Verification items for this drawing (mm, ordinates from the low corner). A direction names the side the tool comes from. Coordinates: 2 decimals unless noted, no trailing zeros. Loops run counter-clockwise (first coordinate to the right, second up) from the corner with the lowest first, then second, coordinate; pieces in that order, holes last.
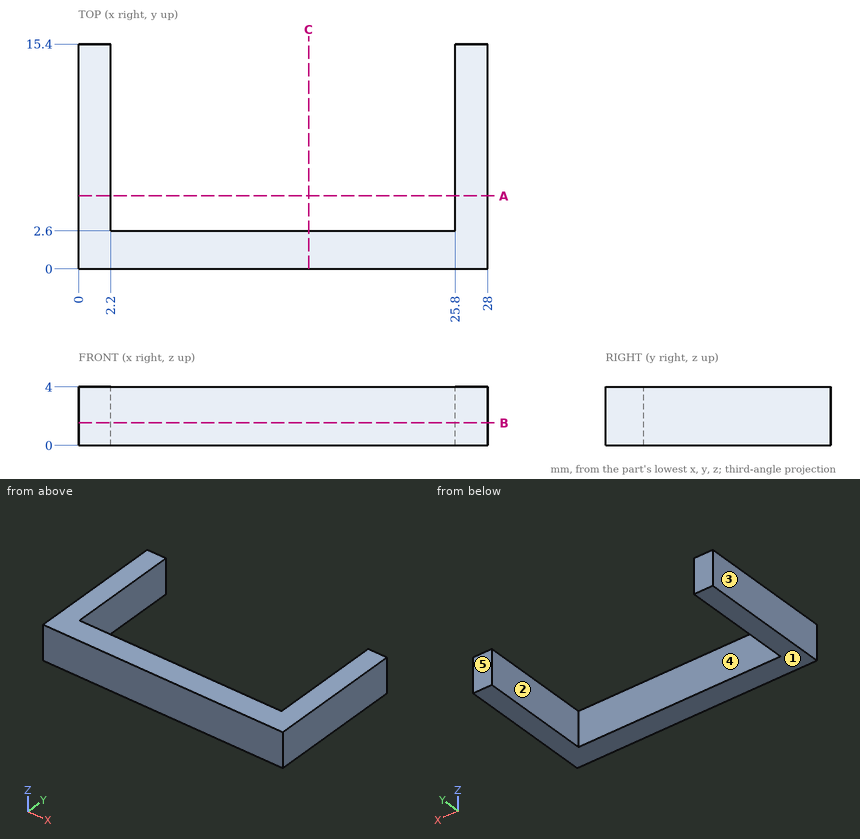
(1) Section check B-B, the plane z = 1.55. Enter the section's corners in (x, y).
(2) Section check C-C, the plane x = 15.75. Enter the section's corners in (y, z).
(3) Set-up check for the marked faces 4 and 5: record each of +Z, -Z, +X, -X, +Y, -Y from which the full face is reachable in a straight line by a thin tool's end or side.
(4) Draft check along X on the marked faces 1, 2 and 3. Enter one of: pulls with the +X half, pulls with the -X half, needs draft (parallel to the pull), parting line crosses it, or undercut.
(5) Section check A-A, the plane y = 5. Enter the section's corners in (x, z).
(6) Scan lines: line 1 along X through (y, z) = (11.5, 0.65); line 2 along Y through (x, z) = (20.25, 0.8). Record each from-to range of solid material in increasing order.
(7) Gauge pin test, flat ends, axial feed: P1, Ø5, axis at x = 19.5, y = 4.5, coming from the +Z side; P2, Ø2, axis at x = 12.5, z = 2, coming from the +Y side; P3, Ø4, axis at x = 5, y = 6, coming from the -Z side. Record the tip position at first contact, or that the pin passes through.
Determined:
1. outline: (0, 0) - (28, 0) - (28, 15.4) - (25.8, 15.4) - (25.8, 2.6) - (2.2, 2.6) - (2.2, 15.4) - (0, 15.4) - close
2. outline: (0, 0) - (2.6, 0) - (2.6, 4) - (0, 4) - close
3. face 4: +Z, -Z, +Y
3. face 5: +Z, -Z, +X, -X, +Y
4. face 1: needs draft
4. face 2: undercut
4. face 3: pulls with the -X half
5. outline: (0, 0) - (2.2, 0) - (2.2, 4) - (0, 4) - close; (25.8, 0) - (28, 0) - (28, 4) - (25.8, 4) - close
6. line 1: x = 0 to 2.2, 25.8 to 28
6. line 2: y = 0 to 2.6
7. P1: stops at z = 4
7. P2: stops at y = 2.6
7. P3: passes through
